Geometry: final body of the model. Coordinates: model frame, mm. A direction names the side the tool comes from. Give positions to 0.01 mm unless a question says otherwise; leave off trailing zeros. Write each loop counter-clockwise with the first axis right and the second up, starting at its lowest first coordinate (ties: lowest second). Pieces come first, ordered by that corner, then holes. Notation, with made-up numbers: M 56.25,67.5 L 114.25,67.5 A20 cw 114.25,90.5 Z; hole C 59.25,-24.5 d5. An arc over 180 degrees is marked long. Use a Markdown table: item, result. Add a question column.
(1) Material intervals for L1, parallel to Y at x = 4, z = 0.55; L2, parallel to Z at x = 19.5, y = 9.5; L3, parallel to Y at x = 51, z = 1.35, sorted ascending.
(2) Cut plane A-A (x = 51). Output: boundary loops of the cut face in (y, z).
(3) Reachability of faces 1 (the flat face through (37, 6, 19)), 2 (the cylindrical face through (30.76, 8.65, 9.89)), 3 (the flat face through (27, 10, 29)) from +Z, -Z, +X, -X, +Y, -Y: full face, straight path, thin tool, end or side. Return the list, or none.
(4) Cut plane D-D (z = 5). Output: boundary loops of the cut face in (x, y).
(5) Draft query along X for faces 4 (the cylindrical face through (51.954, 11.011, 0.986)), 5 (the cylindrical face through (36.737, 6.17, 23.437)), 6 (the flat face through (27, 6, 2)). Return one class per face: released by +X, released by -X, zero draft, split by the parting line, or undercut.
(6) Cut plane B-B (x = 4). Output: boundary loops of the cut face in (y, z), plus the area to 3 significant figures.
(7) Pin query (flat end, axial travel): pin 1 Ø6 at (x, y) = (37.5, 9.5) entering from -Z; pin 2 Ø6 at (x, y) = (41.5, 4) entering from +Z; pin 3 Ø2 at (x, z) = (26, 1) entering from -Y; pin 4 Ø8 at (x, z) = (25, 13.5) entering from +Y. Return the tip coordinate at first contact, or that it passes through.
(8) Cut plane C-C (x = 27.5). Output: boundary loops of the cut face in (y, z), plus the area to 3 significant figures.
```python
from build123d import *

# Parameters (mm, degrees)
SKETCH1_W           = 55
SKETCH1_H           = 20
SKETCH1_R           = 1
BOSS_EXTRUDE1_DEPTH = 2
SKETCH2_R           = 3.526621479
BOSS_EXTRUDE2_DEPTH = 16
SKETCH3_R           = 11
BOSS_EXTRUDE3_DEPTH = 1
SKETCH5_R           = 10
BOSS_EXTRUDE4_DEPTH = 10
FILLET1_R           = 1
FILLET2_R           = 0.5


with BuildPart() as part:
    # Sketch1 → Boss-Extrude1 (new body)
    with BuildSketch(Plane.XY):
        with Locations((27.5, 10)):
            Rectangle(SKETCH1_W, SKETCH1_H)
        with Locations((4, 18)):
            Circle(SKETCH1_R, mode=Mode.SUBTRACT)
        with Locations((4, 2)):
            Circle(SKETCH1_R, mode=Mode.SUBTRACT)
        with Locations((51, 10.710900474)):
            Circle(SKETCH1_R, mode=Mode.SUBTRACT)
    extrude(amount=BOSS_EXTRUDE1_DEPTH)

    # Sketch2 → Boss-Extrude2 (add)
    with BuildSketch(Plane.XY.offset(2)):
        with Locations((27.5, 10)):
            Circle(SKETCH2_R)
    extrude(amount=BOSS_EXTRUDE2_DEPTH)

    # Sketch3 → Boss-Extrude3 (add)
    with BuildSketch(Plane.XY.offset(18)):
        with Locations((27.5, 10)):
            Circle(SKETCH3_R)
    extrude(amount=BOSS_EXTRUDE3_DEPTH)

    # Sketch5 → Boss-Extrude4 (add)
    with BuildSketch(Plane.XY.offset(19)):
        with Locations((27.5, 10)):
            Circle(SKETCH5_R)
    extrude(amount=BOSS_EXTRUDE4_DEPTH)

    # Fillet1
    fillet1_edges = [part.edges().sort_by_distance(p)[0] for p in [
        (17.5, 10, 29),
    ]]
    fillet(fillet1_edges, radius=FILLET1_R)

    # Fillet2
    fillet2_edges = [part.edges().sort_by_distance(p)[0] for p in [
        (16.5, 10, 19),
    ]]
    fillet(fillet2_edges, radius=FILLET2_R)


solid = part.part
```
Answer list:
| question | item | result |
|---|---|---|
| 1 | L1 | 0 to 1, 3 to 17, 19 to 20 |
| 1 | L2 | 0 to 2, 18 to 29 |
| 1 | L3 | 0 to 9.71, 11.71 to 20 |
| 2 | outline | M 0,0 L 9.71,0 L 9.71,2 L 0,2 Z; M 11.71,0 L 20,0 L 20,2 L 11.71,2 Z |
| 3 | face 1 | +Z |
| 3 | face 2 | none |
| 3 | face 3 | +Z, +X, -X, +Y, -Y |
| 4 | outline | C 27.5,10 d7.05 |
| 5 | face 4 | undercut |
| 5 | face 5 | split by the parting line |
| 5 | face 6 | zero draft |
| 6 | outline | M 0,0 L 1,0 L 1,2 L 0,2 Z; M 3,0 L 17,0 L 17,2 L 3,2 Z; M 19,0 L 20,0 L 20,2 L 19,2 Z |
| 6 | area | 32.0 mm² |
| 7 | pin 1 | z = 0 |
| 7 | pin 2 | z = 2 |
| 7 | pin 3 | y = 0 |
| 7 | pin 4 | y = 13.53 |
| 8 | outline | M -1,18 L 6.47,18 L 6.47,2 L 0,2 L 0,0 L 20,0 L 20,2 L 13.53,2 L 13.53,18 L 21,18 L 21,18.5 A0.5 ccw 20.5,19 L 20,19 L 20,28 A1 ccw 19,29 L 1,29 A1 ccw 0,28 L 0,19 L -0.5,19 A0.5 ccw -1,18.5 Z |
| 8 | area | 374 mm² |
